from build123d import *

# Parameters (mm, degrees)
SKETCH_R           = 44.85
PAD_DEPTH          = 4
POCKET_DEPTH       = 4
POLARPATTERN_COUNT = 5
SKETCH003_R        = 5
PAD001_DEPTH       = 6
POCKET001_DEPTH    = 9
FILLET_R           = 2
FILLET001_R        = 4


with BuildPart() as part:
    # Sketch → Pad (new body)
    with BuildSketch(Plane.XY):
        Circle(SKETCH_R)
    extrude(amount=PAD_DEPTH)

    # Sketch002 (on Face2 of Pad) → Pocket (cut)
    with BuildSketch(Plane(origin=(0, 0, 0), x_dir=(1, 0, 0), z_dir=(0, 0, -1))):
        with BuildLine():
            Line((-2.5, 39.821602), (-2.5, 9.682458))
            ThreePointArc((-2.5, 9.682458), (-5.877853, 8.09017), (-8.436023, 5.369685))
            Line((-37.100052, 14.683193), (-8.436023, 5.369685))
            ThreePointArc((-2.5, 39.821602), (-23.452632, 32.279778), (-37.100052, 14.683193))
        make_face()
    pocket = extrude(amount=-POCKET_DEPTH, mode=Mode.SUBTRACT)

    # PolarPattern: Pocket ×5 about axis
    polarpattern_axis = Axis((0, 0, 0), (0, 0, -1))
    for i in range(1, POLARPATTERN_COUNT):
        add(pocket.rotate(polarpattern_axis, i * 360 / POLARPATTERN_COUNT), mode=Mode.SUBTRACT)

    # Sketch003 (on Face3 of PolarPattern) → Pad001 (join)
    with BuildSketch(Plane.XY.offset(4)):
        Circle(SKETCH003_R)
    extrude(amount=PAD001_DEPTH)

    # Sketch004 (on Face25 of Pad001) → Pocket001 (cut)
    with BuildSketch(Plane.XY.offset(10)):
        with BuildLine():
            Line((-1.4, 1.906102), (-1.4, -1.912302))
            ThreePointArc((-1.4, -1.912302), (0, -2.37), (1.4, -1.912302))
            Line((1.4, 1.906102), (1.4, -1.912302))
            ThreePointArc((1.4, 1.906102), (0, 2.365), (-1.4, 1.906102))
        make_face()
    extrude(amount=-POCKET001_DEPTH, mode=Mode.SUBTRACT)

    # Fillet
    fillet_edges = [part.edges().sort_by_distance(p)[0] for p in [
        (-3.668664, 9.302736, 2),
        (3.668664, 9.302736, 2),
        (-7.713749, 6.36381, 2),
        (-9.981108, -0.614403, 2),
        (-8.436023, -5.369685, 2),
        (2.5, -9.682458, 2),
        (8.436023, -5.369685, 2),
        (-2.5, -9.682458, 2),
        (9.981108, -0.614403, 2),
        (7.713749, 6.36381, 2),
    ]]
    fillet(fillet_edges, radius=FILLET_R)

    # Fillet001
    fillet001_edges = [part.edges().sort_by_distance(p)[0] for p in [
        (-38.645137, -9.927911, 2),
        (-25.429093, 30.74689, 2),
        (21.384008, 33.685816, 2),
        (37.100052, -14.683193, 2),
        (-2.5, -39.821602, 2),
        (-37.100052, -14.683193, 2),
        (2.5, -39.821602, 2),
        (25.429093, 30.74689, 2),
        (38.645137, -9.927911, 2),
        (-21.384008, 33.685816, 2),
    ]]
    fillet(fillet001_edges, radius=FILLET001_R)


solid = part.part
CAD build for the part. Positions are in the model's coordinates, mm. A direction names the side the tool comes from. Coordinates: 2 decimals unless noted, no trailing zeros. Loops run counter-clockwise (first coordinate to the right, second up) from the corner with the lowest first, then second, coordinate; pieces in that order, holes last. Notation, with made-up numbers: (-9.5, 16) - (27.5, 16) arc R14 cw to (27.5, 43) - close; hole circle Ø7 at (18.25, 17). An arc over 180 degrees is marked (long way). Use one line per item in the form item = value. Start each with the question number.
1) Band-saw the part on C-C (y = 12.5). Give the cut face in (x, z).
2) Drill centre lines: L1, parallel to Y at x = 17, z = 2; L2, parallel to X at y = 23, z = 2.25; L3, parallel to X at y = 26, z = 1.5. Where is each one in solid material? Low to high. Write a range as from..to.
3) Flat gauge pins, fed straight in: pin 1 (2 mm diameter, centred on y = -21.5, z = 1.5, fed in from +X); pin 2 (3 mm diameter, centred on y = -1, z = 6.5, fed in from +X); pin 3 (5 mm diameter, centred on y = -9.5, z = 5, fed in from +X). Where does each tip first touch, or does it go through?
4) Band-saw the part on A-A (x = 0). Give the cut face in (y, z) (3 decimals), and give its area (3 significant figures).
5) Band-saw the part on B-B (z = 5.25). Give the cut face in (x, y) (3 decimals).
6) Band-saw the part on D-D (x = -31). Give the cut face in (y, z), and give its area (3 significant figures).
7) Two-plate mould, pull along X, no slides. Class faces 1 (the face through (-35.59, -27.29, 1.97)), 2 (the face through (-8.62, -5.8, 2.03)), 3 (the face through (-0.02, -2.37, 5.56)), 4 (the face through (2, 0, 10)): +X half, -X half, draft (parallel to the pull), parting line (faces both ways), or undercut.
8) Tool access for faces 5 (the face through (0, 0, 1)), 6 (the face through (9.5, 3.12, 1.97)): list every direction of +Z, -Z, +X, -X, +Y, -Y with a clear straight run to the whole face (end or side of a thin tool).
Check values:
q1.outline = (-43.07, 0) - (-37.89, 0) - (-37.89, 4) - (-43.07, 4) - close; (-12.17, 0) - (-5.99, 0) - (-5.99, 4) - (-12.17, 4) - close; (5.99, 0) - (12.17, 0) - (12.17, 4) - (5.99, 4) - close; (37.89, 0) - (43.07, 0) - (43.07, 4) - (37.89, 4) - close
q2.L1 = -41.5..-36.1, -8.15..-2.89, 19.15..27.65, 36.1..41.5
q2.L2 = -38.5..-32.6, -19.8..-13.62, 13.62..19.8, 32.6..38.5
q2.L3 = -36.54..-30.27, -21.98..-15.8, 15.8..21.98, 30.27..36.54
q3.pin_1 = 39.89
q3.pin_2 = 5
q3.pin_3 = 44.27
q4.outline = (-44.85, 0) - (10, 0) - (10, 4) - (5, 4) - (5, 10) - (2.365, 10) - (2.365, 1) - (-2.37, 1) - (-2.37, 10) - (-5, 10) - (-5, 4) - (-44.85, 4) - close; (39.9, 0) - (44.85, 0) - (44.85, 4) - (39.9, 4) - close
q4.area = 257 mm2
q5.outline = circle Ø10 at (0, 0); hole (-1.4, -1.912) arc R2.37 ccw to (1.4, -1.912) - (1.4, 1.906) arc R2.365 ccw to (-1.4, 1.906) - close
q6.outline = (-32.41, 0) - (-25.12, 0) - (-25.12, 4) - (-32.41, 4) - close; (-12.7, 0) - (-7.44, 0) - (-7.44, 4) - (-12.7, 4) - close; (25.12, 0) - (32.41, 0) - (32.41, 4) - (25.12, 4) - close
q6.area = 79.4 mm2
q7.face_1 = parting line
q7.face_2 = undercut
q7.face_3 = undercut
q7.face_4 = draft
q8.face_5 = +Z
q8.face_6 = +Z, -Z
